Input: part model. Units: mm. Frame: model coordinates. Coordinates: 2 decimals unless noted, no trailing zeros. Order: outer loops, then holes, each group sorted by start corner. A loop starts at its lowest first (then second) coordinate and runs counter-clockwise, first axis right, second up. Notation, with made-up numbers: (5, -31) -> (36, -31) arc R26 ccw to (36, -5) -> close; hole circle Ø1 at (82.5, 25). An arc over 180 degrees is marked (long way). Use one line per item in the form item = value. Start each with the question number.
1) Pin query (flat end, axial travel): pin 1 (0.9 mm diameter, centred on y = 0.5, z = 22, fed in from +X); pin 2 (1.1 mm diameter, centred on x = -11, y = 3, fed in from +Z); pin 3 (1.9 mm diameter, centred on x = -4, y = 2, fed in from -Z). Return the tip coordinate at first contact, or that it passes through.
2) Section query B-B on y = 3.15. Output: boundary loops of the cut face in (x, z).
3) Ray query, line 1 along Y through (x, z) = (-20, 12); line 2 along Z through (x, y) = (-8, 2.85). Return the intervals inside material, ascending.
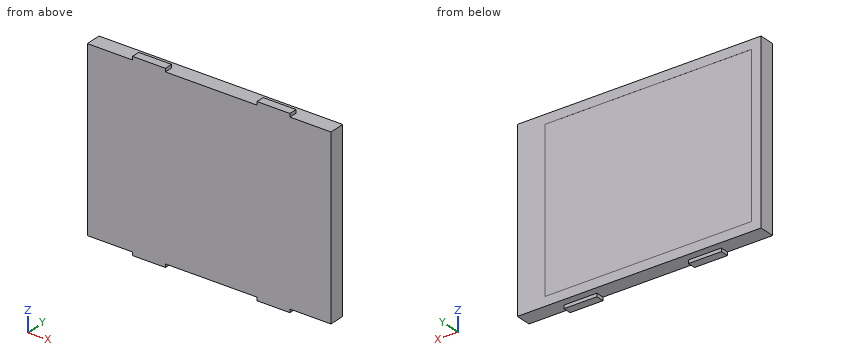
from build123d import *

# Parameters (mm, degrees)
SKETCH1_W           = 59.26
SKETCH1_H           = 42.72
BOSS_EXTRUDE1_DEPTH = 3.8
SKETCH2_W           = 8
SKETCH2_H           = 2
BOSS_EXTRUDE2_DEPTH = 0.8
SKETCH3_W           = 8
SKETCH3_H           = 2
BOSS_EXTRUDE3_DEPTH = 0.8
SKETCH4_W           = 50.2
SKETCH4_H           = 38.3
CUT_EXTRUDE1_DEPTH  = 0.01


with BuildPart() as part:
    # Sketch1 → Boss-Extrude1 (new body)
    with BuildSketch(Plane(origin=(0, 0, 0), x_dir=(1, 0, 0), z_dir=(0, 1, 0))):
        Rectangle(SKETCH1_W, SKETCH1_H)
    extrude(amount=BOSS_EXTRUDE1_DEPTH)

    # Sketch2 → Boss-Extrude2 (add)
    with BuildSketch(Plane.XY.offset(21.36)):
        with Locations((-14.63, 1)):
            Rectangle(SKETCH2_W, SKETCH2_H)
        with Locations((15.63, 1)):
            Rectangle(SKETCH2_W, SKETCH2_H)
    extrude(amount=BOSS_EXTRUDE2_DEPTH)

    # Sketch3 → Boss-Extrude3 (add)
    with BuildSketch(Plane(origin=(0, 0, -21.36), x_dir=(-1, 0, 0), z_dir=(0, 0, -1))):
        with Locations((14.63, 1)):
            Rectangle(SKETCH3_W, SKETCH3_H)
        with Locations((-15.63, 1)):
            Rectangle(SKETCH3_W, SKETCH3_H)
    extrude(amount=BOSS_EXTRUDE3_DEPTH)

    # Sketch4 → Cut-Extrude1 (cut)
    with BuildSketch(Plane(origin=(0, 3.8, 0), x_dir=(1, 0, 0), z_dir=(0, 1, 0))):
        with Locations((-2.23, 0)):
            Rectangle(SKETCH4_W, SKETCH4_H)
    extrude(amount=-CUT_EXTRUDE1_DEPTH, mode=Mode.SUBTRACT)


solid = part.part
Answers below:
q1.pin_1 = 19.63
q1.pin_2 = 21.36
q1.pin_3 = -21.36
q2.outline = (-29.63, -21.36) -> (29.63, -21.36) -> (29.63, 21.36) -> (-29.63, 21.36) -> close
q3.line_1 = 0 to 3.79
q3.line_2 = -21.36 to 21.36
